Verification items for the finished model (mm, model axes). A direction names the side the tool comes from. Round coordinates to 2 decimals unless told otherwise and drop trailing zeros. Write each loop counter-clockwise with the first axis right and the second up, starting at its lowest first coordinate (ties: lowest second). Pieces come first, ordered by that corner, then holes. Notation, with made-up numbers: (70.25, 0.5) -> (79.25, 0.5) arc R12 ccw to (79.25, 13.5) -> close; hole circle Ø4 at (87, -15). An arc over 180 degrees is marked (long way). Answer as a JSON object with one key per item and string values. Group by question number.
(1) Sectioned sample at C-C on x = -6.25. Record the cut outline in (y, z).
(2) Draft check along X on faces 1 (the face through (-7.5, -1, 0)), 2 (the face through (0, 1, 1.75)), 3 (the face through (-2.2, 62.3, -0.6)). Enter one of: released by +X, released by -X, zero draft, split by the parting line, or undercut.
(3) Scan lines: L1, parallel to Y at x = 0.5, z = 0.5; L2, parallel to Z at x = 2.5, y = 61.5. Record each from-to range of solid material in increasing order. Write a range as from..to.
(4) Set-up check for faces 4 (the face through (0, 1, -1.75)), 5 (the face through (3.8, 62.3, -0.6)): record each of +Z, -Z, +X, -X, +Y, -Y from which the full face is reachable in a straight line by a thin tool's end or side.
(5) Gauge pin test, flat end, axial feed: pin 1 Ø1 at (x, z) = (0, 0) entering from +Y. Record the tip position at first contact, or that the pin passes through.
(6) Sectioned sample at B-B on z = 0. Record the cut outline in (x, y).
(7) Sectioned sample at A-A on y = 52.5. Record the cut outline in (x, z), and give its area (3 significant figures).
```python
from build123d import *

# Parameters (mm, degrees)
F0_W     = 15
F0_H     = 100
F1_DEPTH = 1.75
F2_R     = 1
F3_DEPTH = 25


with BuildPart() as f1:
    # F0 (on Top) → F1 (new body, symmetric)
    with BuildSketch(Plane.XY):
        Rectangle(F0_W, F0_H)
    extrude(amount=F1_DEPTH, both=True)

    # F2 (on face) → F3 (join)
    with BuildSketch(Plane(origin=(0, 50, 0), x_dir=(-1, 0, 0), z_dir=(0, 1, 0))):
        with Locations((3, 0)):
            Circle(F2_R)
        with Locations((-3, 0)):
            Circle(F2_R)
    extrude(amount=F3_DEPTH)


solid = f1.part
```
Computed values:
{
 "1": {"outline": "(-50, -1.75) -> (50, -1.75) -> (50, 1.75) -> (-50, 1.75) -> close"},
 "2": {"face 1": "released by -X", "face 2": "zero draft", "face 3": "undercut"},
 "3": {"L1": "-50..50", "L2": "-0.87..0.87"},
 "4": {"face 4": "-Z, +X, -X, +Y, -Y", "face 5": "+Y"},
 "5": {"pin 1": "y = 50"},
 "6": {"outline": "(-7.5, -50) -> (7.5, -50) -> (7.5, 50) -> (4, 50) -> (4, 75) -> (2, 75) -> (2, 50) -> (-2, 50) -> (-2, 75) -> (-4, 75) -> (-4, 50) -> (-7.5, 50) -> close"},
 "7": {"outline": "circle Ø2 at (-3, 0); circle Ø2 at (3, 0)", "area": "6.28 mm2"}
}
